Work out the finished part from the listing and answer in its coordinate system (mm). A direction names the side the tool comes from. Give positions to 0.01 mm unless a question says otherwise; leave off trailing zeros. Loops run counter-clockwise (first coordinate to the right, second up) from the corner with the lowest first, then second, coordinate; pieces in that order, holes last. Notation, with made-up numbers: M 57,53.25 L 116,53.25 A27 cw 116,80.25 Z; hole C 85.5,55 d4. An arc over 180 degrees is marked long. Use a Markdown table: item, result.
```python
from build123d import *

# Parameters (mm, degrees)
SKETCH_1_W             = 30
SKETCH_1_H             = 30
SKETCH_1_W_2           = 24
SKETCH_1_H_2           = 24
EXTRUDE_1_DEPTH        = 729
HOLE_WIZARD_7_0_7_1_D  = 7
PATTERN_LINEAR_1_COUNT = 2
PATTERN_LINEAR_1_PITCH = 678.25


with BuildPart() as part:
    # 草图1 → 拉伸1 (new body)
    with BuildSketch(Plane.XY):
        with Locations((15, -15)):
            Rectangle(SKETCH_1_W, SKETCH_1_H)
        with Locations((15, -15)):
            Rectangle(SKETCH_1_W_2, SKETCH_1_H_2, mode=Mode.SUBTRACT)
    extrude(amount=EXTRUDE_1_DEPTH)

    # Ø7.0 (7) 直径孔1 (through all)
    with Locations(Plane(origin=(30, 0, 0), x_dir=(0, 0, -1), z_dir=(1, 0, 0))):
        with Locations((-718, -15), (-690, -15)):
            hole_wizard_7_0_7_1 = Hole(HOLE_WIZARD_7_0_7_1_D / 2)

    # 阵列(线性)1: Ø7.0 (7) 直径孔1 ×2
    with Locations(*[(0, 0, -i * PATTERN_LINEAR_1_PITCH) for i in range(1, PATTERN_LINEAR_1_COUNT)]):
        add(hole_wizard_7_0_7_1, mode=Mode.SUBTRACT)


solid = part.part
```
(1) Consider probe 1 along X at (y, z) = (-26.5, 277); probe 2 along Y at (x, z) = (28, 11.75); probe 3 along Y at (x, z) = (21, 323). Determine where each line is inside the solid, lowest interval first. Write a range as [from, to].
Entries:
| item | result |
|---|---|
| probe 1 | x = [0, 3], [27, 30] |
| probe 2 | y = [-30, -18.5], [-11.5, 0] |
| probe 3 | y = [-30, -27], [-3, 0] |
(2) The mould has two halves that part along X. Classify faces 3 (the flat face through (28, -15, 729)), 4 (the flat face through (0, -15, 359)), 5 (the flat face through (30, -15, 359)), 6 (the flat face through (3, -15, 359)): released by +X, released by -X, zero draft, split by the parting line, or undercut.
Entries:
| item | result |
|---|---|
| face 3 | zero draft |
| face 4 | released by -X |
| face 5 | released by +X |
| face 6 | undercut |
(3) A cutting plane is placed at B-B (z = 332.5). Write down the section's boundary in (x, y), and give its area (3 significant figures).
Entries:
| item | result |
|---|---|
| outline | M 0,-30 L 30,-30 L 30,0 L 0,0 Z; hole M 3,-27 L 27,-27 L 27,-3 L 3,-3 Z |
| area | 324 mm² |
(4) Which of the six approach directions +Z, -Z, +X, -X, +Y, -Y give full straight-line access (tool end or side, diameter ignored) to faces 1 (the flat face through (15, 0, 359)), 2 (the flat face through (27, -15, 359))?
Entries:
| item | result |
|---|---|
| face 1 | +Z, -Z, +X, -X, +Y |
| face 2 | +Z, -Z |
(5) Given P1, Ø8, axis at x = 6.5, y = -21, coming from the +Z side, flat-ended and moving along its own axis, determine where the tip first touches the part or whether it passes through.
Entries:
| item | result |
|---|---|
| P1 | stops at z = 729 |
(6) A cutting plane is placed at A-A (x = 15.75). Write down the section's boundary in (y, z).
Entries:
| item | result |
|---|---|
| outline | M -30,0 L -27,0 L -27,729 L -30,729 Z; M -3,0 L 0,0 L 0,729 L -3,729 Z |
